from build123d import *

# Parameters (mm, degrees)
SKETCH_R  = 2.75
PAD_DEPTH = 40


with BuildPart() as part:
    # Sketch → Pad (new body)
    with BuildSketch(Plane.XY):
        with BuildLine():
            ThreePointArc((-8.5, 10), (-9.56066, 9.56066), (-10, 8.5))
            Line((-10, 8.5), (-10, 4.5))
            Line((-10, 4.5), (-8.5, 3))
            Line((-8.5, 3), (-8.5, 7.43934))
            Line((-8.5, 7.43934), (-4.5, 3.43934))
            Line((-4.5, 3.43934), (-4.5, -3.43934))
            Line((-4.5, -3.43934), (-8.5, -7.43934))
            Line((-8.5, -7.43934), (-8.5, -3))
            Line((-8.5, -3), (-10, -4.5))
            Line((-10, -4.5), (-10, -8.5))
            ThreePointArc((-10, -8.5), (-9.56066, -9.56066), (-8.5, -10))
            Line((-8.5, -10), (-4.5, -10))
            Line((-4.5, -10), (-3, -8.5))
            Line((-3, -8.5), (-7.43934, -8.5))
            Line((-7.43934, -8.5), (-3.43934, -4.5))
            Line((-3.43934, -4.5), (3.43934, -4.5))
            Line((3.43934, -4.5), (7.43934, -8.5))
            Line((7.43934, -8.5), (3, -8.5))
            Line((3, -8.5), (4.5, -10))
            Line((4.5, -10), (8.5, -10))
            ThreePointArc((8.5, -10), (9.56066, -9.56066), (10, -8.5))
            Line((10, -8.5), (10, -4.5))
            Line((10, -4.5), (8.5, -3))
            Line((8.5, -3), (8.5, -7.43934))
            Line((8.5, -7.43934), (4.5, -3.43934))
            Line((4.5, -3.43934), (4.5, 3.43934))
            Line((4.5, 3.43934), (8.5, 7.43934))
            Line((8.5, 7.43934), (8.5, 3))
            Line((8.5, 3), (10, 4.5))
            Line((10, 4.5), (10, 8.5))
            ThreePointArc((10, 8.5), (9.56066, 9.56066), (8.5, 10))
            Line((8.5, 10), (4.5, 10))
            Line((4.5, 10), (3, 8.5))
            Line((3, 8.5), (7.43934, 8.5))
            Line((7.43934, 8.5), (3.43934, 4.5))
            Line((-3.43934, 4.5), (3.43934, 4.5))
            Line((-7.43934, 8.5), (-3.43934, 4.5))
            Line((-3, 8.5), (-7.43934, 8.5))
            Line((-4.5, 10), (-3, 8.5))
            Line((-8.5, 10), (-4.5, 10))
        make_face()
        Circle(SKETCH_R, mode=Mode.SUBTRACT)
    extrude(amount=PAD_DEPTH)


solid = part.part
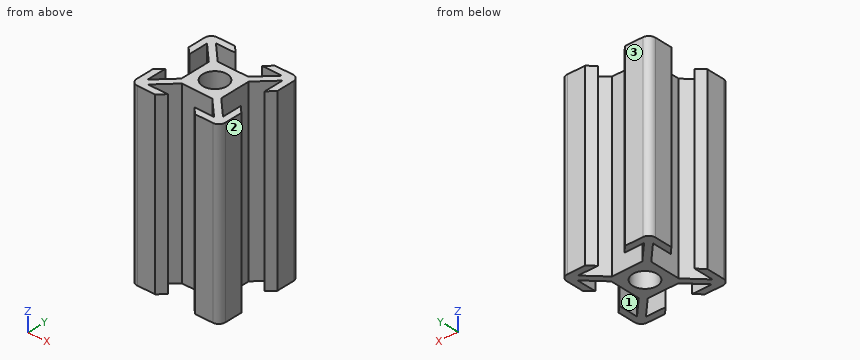
Work out the finished part from the listing and answer in its coordinate system (mm). Face numbers are marked on the shaded views. Coordinates: 2 decimals unless noted, no trailing zeros. Write each loop counter-clockwise with the first axis right and the second up, starting at its lowest first coordinate (ties: lowest second). Pieces come first, ordered by that corner, then holes. Notation, with made-up numbers: M 48,-30 L 106,-30 A12 ccw 106,-26 Z; hole C -5,12.5 d6. An arc over 180 degrees is marked long. Answer as CSV lines item,"result". Start each with the question number.
Item 1: Determine the mould class of the marked faces 1, 2 and 3 for opening direction Y: released by +Y, released by -Y, zero draft, split by the parting line, or undercut.
Item 2: Section A-A on y = 0 is taken. Write down the section's boundary in (x, z).
Item 3: Section D-D on x = -5 is taken. Write down the section's boundary in (y, z).
Item 4: Flat-ended cylindrical pins translate along their axes: P1, Ø5.5, axis at x = 1.5, z = 13.5, coming from the -Y side; P2, Ø3.5, axis at x = 0, z = 18, coming from the +Y side; P3, Ø4.5, axis at x = 0, y = 0, coming from the +Z side; P4, Ø5.5, axis at y = 0, z = 25.5, coming from the -X side. Find the tip coordinate at first contact, or state that the pin passes through.
Item 5: Section C-C on y = 7 is taken. Write down the section's boundary in (x, z), and give its area (3 significant figures).
Item 6: Consider L1, parallel to Y at x = 0, z = 13; L2, parallel to Y at x = 3.5, z = 32; L3, parallel to Y at x = 4, z = 38. Determine where each line is inside the solid, lowest interval first.
Checks:
1,face 1,"undercut"
1,face 2,"zero draft"
1,face 3,"released by +Y"
2,outline,"M -4.5,0 L -2.75,0 L -2.75,40 L -4.5,40 Z; M 2.75,0 L 4.5,0 L 4.5,40 L 2.75,40 Z"
3,outline,"M -10,0 L -8.5,0 L -8.5,40 L -10,40 Z; M -6.06,0 L -3.94,0 L -3.94,40 L -6.06,40 Z; M 3.94,0 L 6.06,0 L 6.06,40 L 3.94,40 Z; M 8.5,0 L 10,0 L 10,40 L 8.5,40 Z"
4,P1,"stops at y = -9.75"
4,P2,"stops at y = 4.5"
4,P3,"passes through"
4,P4,"stops at x = -4.5"
5,outline,"M -10,0 L -8.5,0 L -8.5,40 L -10,40 Z; M -8.06,0 L -5.94,0 L -5.94,40 L -8.06,40 Z; M 5.94,0 L 8.06,0 L 8.06,40 L 5.94,40 Z; M 8.5,0 L 10,0 L 10,40 L 8.5,40 Z"
5,area,"290 mm²"
6,L1,"y = -4.5 to -2.75, 2.75 to 4.5"
6,L2,"y = -9 to -8.5, -4.56 to 4.56, 8.5 to 9"
6,L3,"y = -9.5 to -8.5, -5.06 to 5.06, 8.5 to 9.5"
